from build123d import *

# Parameters (mm, degrees)
FILLET3_R           = 1
CUT_EXTRUDE6_START  = -3.94
CUT_EXTRUDE6_DEPTH  = 3.94
FILLET5_R           = 1
CUT_EXTRUDE7_DEPTH  = 10.94
SKETCH14_W          = 7.26
SKETCH14_H          = 7.85
BOSS_EXTRUDE2_DEPTH = 6.47
CUT_EXTRUDE16_DEPTH = 16.47
SKETCH19_R          = 2.891830788
SKETCH19_R_2        = 2.68
CUT_EXTRUDE20_DEPTH = 1.34
CUT_EXTRUDE21_START = -1.34
SKETCH21_R          = 2.89
SKETCH21_R_2        = 2.68
CUT_EXTRUDE21_DEPTH = 1.34
SKETCH23_R          = 2.68
CUT_EXTRUDE22_DEPTH = 21.34


with BuildPart() as part:
    # Sketch1 → Revolve1 (revolve)
    with BuildSketch(Plane(origin=(0, 0, 0), x_dir=(1, 0, 0), z_dir=(0, 1, 0)), mode=Mode.PRIVATE) as revolve1_sk:
        Polygon((0, 5.74), (10.635, 5.74), (10.635, 3.78), (10.285, 3.78), (10.285, 0.82), (10.89, 0.82), (10.89, -0.45), (9.01, -0.45), (9.01, 0), (0, 0), align=None)
    revolve(revolve1_sk.sketch.rotate(Axis((0, 0, -20.772745763), (0, 0, 1)), 180), axis=Axis((0, 0, -20.772745763), (0, 0, 1)))

    # Fillet3
    # the kernel refuses this fillet: 1 mm, written as the material it takes off along each edge
    with BuildSketch(Plane(origin=(0, 0, -3.78), x_dir=(-1, 0, 0), z_dir=(0, 1, 0))) as fillet3_piece_1:
        with BuildLine():
            CenterArc((9.635, -0.759934208), FILLET3_R, 0, 49.458398126)
            Line((10.285, 0), (10.298, 0.015198684))
            ThreePointArc((10.298, 0.015198684), (10.46, 0.02), (10.635, 0.02))
            Line((10.635, 0.02), (10.655, 0))
            Line((10.655, 0), (10.655, -0.759934208))
            Line((10.655, -0.759934208), (10.635, -0.759934208))
        make_face()
    revolve(axis=Axis((0, 0, -3.78), (0, 0, 1)), mode=Mode.SUBTRACT)
    with BuildSketch(Plane(origin=(0, 0, -5.74), x_dir=(-1, 0, 0), z_dir=(0, 1, 0))) as fillet3_piece_2:
        with BuildLine():
            CenterArc((10.635 - FILLET3_R, FILLET3_R), FILLET3_R, 270, 90)
            Line((10.635, FILLET3_R), (10.635 + FILLET3_R * 0.02, FILLET3_R))
            Line((10.635 + FILLET3_R * 0.02, FILLET3_R), (10.635 + FILLET3_R * 0.02, -FILLET3_R * 0.02))
            Line((10.635 + FILLET3_R * 0.02, -FILLET3_R * 0.02), (10.635 - FILLET3_R, -FILLET3_R * 0.02))
            Line((10.635 - FILLET3_R, -FILLET3_R * 0.02), (10.635 - FILLET3_R, 0))
        make_face()
    revolve(axis=Axis((0, 0, -5.74), (0, 0, 1)), mode=Mode.SUBTRACT)
    with BuildSketch(Plane(origin=(0, 0, -0.82), x_dir=(-1, 0, 0), z_dir=(0, 1, 0))) as fillet3_piece_3:
        with BuildLine():
            CenterArc((9.89, 0.91868112), FILLET3_R, 293.265974062, 66.734025938)
            Line((10.89, 0.91868112), (10.91, 0.91868112))
            Line((10.91, 0.91868112), (10.91, 0))
            Line((10.91, 0), (10.89, -0.02))
            ThreePointArc((10.89, -0.02), (10.5875, -0.02), (10.2929, -0.018373622))
            Line((10.2929, -0.018373622), (10.285, 0))
        make_face()
    revolve(axis=Axis((0, 0, -0.82), (0, 0, 1)), mode=Mode.SUBTRACT)

    # Sketch13 → Cut-Extrude6 (cut)
    with BuildSketch(Plane.XY.offset(CUT_EXTRUDE6_START)):
        with BuildLine():
            Line((-5.63, -5.63), (-5.63, 5.63))
            Line((-5.63, 5.63), (-5.63, 7.034429614))
            ThreePointArc((-5.63, 7.034429614), (-9.01, 0), (-5.63, -7.034429614))
            Line((-5.63, -7.034429614), (-5.63, -5.63))
        make_face()
        with BuildLine():
            Line((5.63, -5.63), (-5.63, -5.63))
            Line((-5.63, -5.63), (-5.63, -7.034429614))
            ThreePointArc((-5.63, -7.034429614), (0, -9.01), (5.63, -7.034429614))
            Line((5.63, -7.034429614), (5.63, -5.63))
        make_face()
        with BuildLine():
            Line((5.63, 7.034429614), (5.63, 5.63))
            Line((5.63, 5.63), (5.63, -5.63))
            Line((5.63, -5.63), (5.63, -7.034429614))
            ThreePointArc((5.63, -7.034429614), (8.121157553, -3.902166065), (9.01, 0))
            ThreePointArc((9.01, 0), (8.121157553, 3.902166065), (5.63, 7.034429614))
        make_face()
        with BuildLine():
            Line((-5.63, 7.034429614), (-5.63, 5.63))
            Line((-5.63, 5.63), (5.63, 5.63))
            Line((5.63, 5.63), (5.63, 7.034429614))
            ThreePointArc((5.63, 7.034429614), (0, 9.01), (-5.63, 7.034429614))
        make_face()
    extrude(amount=CUT_EXTRUDE6_DEPTH, mode=Mode.SUBTRACT)

    # Fillet5
    fillet5_edges = [part.edges().sort_by_distance(p)[0] for p in [
        (-5.63, 5.63, -1.97),
        (-5.63, -5.63, -1.97),
        (5.63, -5.63, -1.97),
        (5.63, 5.63, -1.97),
    ]]
    fillet(fillet5_edges, radius=FILLET5_R)

    # 3DSketch1 → Cut-Extrude7 (cut)
    with BuildSketch(Plane(origin=(-4.37, -4.37, 0), x_dir=(0.7071067811865485, 0.7071067811865467, 0), z_dir=(0, 0, -1))):
        with BuildLine():
            Line((0.707106781, 0.707106781), (5.473006486, 5.473006486))
            ThreePointArc((5.473006486, 5.473006486), (6.180113268, 5.765899705), (6.887220049, 5.473006486))
            Line((6.887220049, 5.473006486), (11.653119754, 0.707106781))
            ThreePointArc((11.653119754, 0.707106781), (11.946012973, 0), (11.653119754, -0.707106781))
            Line((11.653119754, -0.707106781), (6.887220049, -5.473006486))
            ThreePointArc((6.887220049, -5.473006486), (6.180113268, -5.765899705), (5.473006486, -5.473006486))
            Line((5.473006486, -5.473006486), (0.707106781, -0.707106781))
            ThreePointArc((0.707106781, -0.707106781), (0.414213562, 0), (0.707106781, 0.707106781))
        make_face()
    extrude(amount=CUT_EXTRUDE7_DEPTH, mode=Mode.SUBTRACT)

    # Sketch14 → Boss-Extrude2 (add)
    with BuildSketch(Plane(origin=(0, 0, -5.74), x_dir=(-1, 0, 0), z_dir=(0, 0, -1))):
        with Locations((-8, -0.555)):
            Rectangle(SKETCH14_W, SKETCH14_H)
        with Locations((8, -0.555)):
            Rectangle(SKETCH14_W, SKETCH14_H)
    extrude(amount=BOSS_EXTRUDE2_DEPTH)

    # Sketch16 → Cut-Extrude16 (cut)
    with BuildSketch(Plane.XZ.offset(4.48)):
        with BuildLine():
            ThreePointArc((-4.99, -8.975), (-8, -11.985), (-11.01, -8.975))
            Line((-11.01, -8.975), (-11.01, -5.74))
            Line((-11.01, -5.74), (-11.63, -5.74))
            Line((-11.63, -5.74), (-11.63, -12.21))
            Line((-11.63, -12.21), (-4.37, -12.21))
            Line((-4.37, -12.21), (-4.37, -5.74))
            Line((-4.37, -5.74), (-4.99, -5.74))
            Line((-4.99, -5.74), (-4.99, -8.975))
        make_face()
        with BuildLine():
            ThreePointArc((11.01, -8.975), (8, -11.985), (4.99, -8.975))
            Line((4.99, -8.975), (4.99, -5.74))
            Line((4.99, -5.74), (4.37, -5.74))
            Line((4.37, -5.74), (4.37, -12.21))
            Line((4.37, -12.21), (11.63, -12.21))
            Line((11.63, -12.21), (11.63, -5.74))
            Line((11.63, -5.74), (11.01, -5.74))
            Line((11.01, -5.74), (11.01, -8.975))
        make_face()
    extrude(amount=-CUT_EXTRUDE16_DEPTH, mode=Mode.SUBTRACT)

    # Sketch19 → Cut-Extrude20 (cut)
    # profile 1 of 2: a face of its own
    with BuildSketch(Plane(origin=(0, 3.37, 0), x_dir=(1, 0, 0), z_dir=(0, 1, 0))):
        with Locations(Location((-8, 8.975, 0), (0, 0, 180))):
            Circle(SKETCH19_R)
        with Locations(Location((-8, 8.975, 0), (0, 0, 180))):
            Circle(SKETCH19_R_2, mode=Mode.SUBTRACT)
    # profile 2 of 2: a face of its own
    with BuildSketch(Plane(origin=(0, 3.37, 0), x_dir=(1, 0, 0), z_dir=(0, 1, 0))):
        with Locations((8, 8.975)):
            Circle(SKETCH19_R)
        with Locations((8, 8.975)):
            Circle(SKETCH19_R_2, mode=Mode.SUBTRACT)
    extrude(amount=-CUT_EXTRUDE20_DEPTH, mode=Mode.SUBTRACT)

    # Sketch21 → Cut-Extrude21 (cut)
    # profile 1 of 2: a face of its own
    with BuildSketch(Plane.XZ.offset(4.48).offset(CUT_EXTRUDE21_START)):
        with Locations(Location((-8, -8.975, 0), (0, 0, 270))):
            Circle(SKETCH21_R)
        with Locations(Location((-8, -8.975, 0), (0, 0, 180))):
            Circle(SKETCH21_R_2, mode=Mode.SUBTRACT)
    # profile 2 of 2: a face of its own
    with BuildSketch(Plane.XZ.offset(4.48).offset(CUT_EXTRUDE21_START)):
        with Locations(Location((8, -8.975, 0), (0, 0, 90))):
            Circle(SKETCH21_R)
        with Locations((8, -8.975)):
            Circle(SKETCH21_R_2, mode=Mode.SUBTRACT)
    extrude(amount=CUT_EXTRUDE21_DEPTH, mode=Mode.SUBTRACT)

    # Sketch23 → Cut-Extrude22 (cut)
    with BuildSketch(Plane(origin=(0, 3.37, 0), x_dir=(1, 0, 0), z_dir=(0, 1, 0))):
        with Locations(Location((-8, 8.975, 0), (0, 0, 180))):
            Circle(SKETCH23_R)
        with Locations(Location((8, 8.975, 0), (0, 0, 270))):
            Circle(SKETCH23_R)
    extrude(amount=-CUT_EXTRUDE22_DEPTH, mode=Mode.SUBTRACT)


solid = part.part
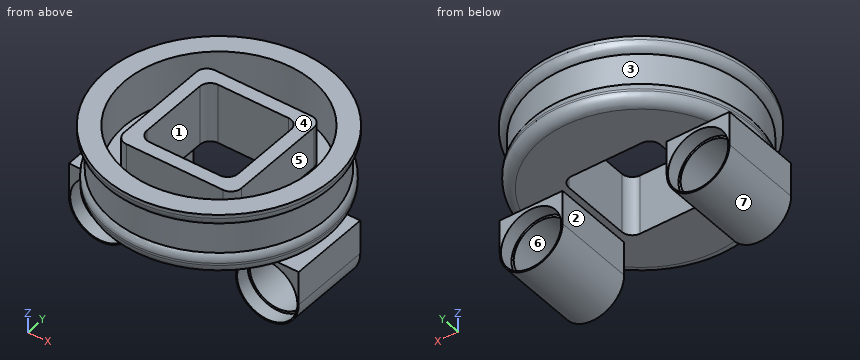
Here's how the part is built. I have some questions about the finished solid (model axes, mm). Face numbers are marked on the shaded views. A direction names the side the tool comes from. Coordinates: 2 decimals unless noted, no trailing zeros. Order: outer loops, then holes, each group sorted by start corner. A loop starts at its lowest first (then second) coordinate and runs counter-clockwise, first axis right, second up. Notation, with made-up numbers: M 76.25,63 L 134.25,63 A28 cw 134.25,101 Z; hole C 66.25,-22.75 d1. An arc over 180 degrees is marked long. Answer as CSV lines item,"result".
Item 1: For pin 1 (4 mm diameter, centred on x = 6, z = -10, fed in from -Y); pin 2 (1.2 mm diameter, centred on x = 1, z = -2.5, fed in from -Y); pin 3 (1.5 mm diameter, centred on y = -2.5, z = -2.5, fed in from -X) (3 decimals); pin 4 (3 mm diameter, centred on x = -7.5, z = -9, fed in from -Y), each with a flat end and sliding along its axis, tell me the tip position at first contact or that it passes through.
Results found:
pin 1,"y = -4.48"
pin 2,"y = -10.28"
pin 3,"x = -10.135"
pin 4,"through"
Item 2: If I drill on line 1 (Y direction, x = 0, z = -1.6) (3 decimals); line 2 (X direction, y = 0.25, z = -4.5); line 3 (X direction, y = 3.5, z = -2), over which ranges is the centre line in solid material (lowest first)?
Results found:
line 1,"-10.285 to -9.01, -5.63 to -4.37, 4.37 to 5.63, 9.01 to 10.285"
line 2,"-10.63 to -4.37, 4.37 to 10.63"
line 3,"-9.67 to -8.3, -5.63 to -4.36, 4.36 to 5.63, 8.3 to 9.67"
Item 3: Imagine slicing it at A-A on z = -1.5. Write out the boundary of the cut face in (x, y) (3 decimals), plus the area to 3 significant figures.
Results found:
outline,"C 0,0 d20.57; M -5.63,-4.63 A1 ccw -4.63,-5.63 L 4.63,-5.63 A1 ccw 5.63,-4.63 L 5.63,4.63 A1 ccw 4.63,5.63 L -4.63,5.63 A1 ccw -5.63,4.63 Z; hole C 0,0 d18.02; hole M -4.37,-3.37 A1 ccw -3.37,-4.37 L 3.37,-4.37 A1 ccw 4.37,-3.37 L 4.37,3.37 A1 ccw 3.37,4.37 L -3.37,4.37 A1 ccw -4.37,3.37 Z"
area,"128 mm2"
Item 4: We'd pull the mould along Z, two halves only. Please class the marked faces 5, 6 and 7: +Z half, -Z half, draft (parallel to the pull), parting line (faces both ways), or undercut.
Results found:
face 5,"draft"
face 6,"undercut"
face 7,"-Z half"
Item 5: On a 3-axis mill with a long thin cutter (end or side, diameter ignored), from which of +Z, -Z, +X, -X, +Y, -Y can I reach the whole of each face in a straight line? I mean the marked faces 1, 2, 3 and 4. Say none if no direction works.
Results found:
face 1,"+Z, -Z"
face 2,"-Z, +Y, -Y"
face 3,"none"
face 4,"+Z"
